from build123d import *

# Parameters (mm, degrees)
F1_DEPTH      = 210
F0_W          = 7
F0_H          = 48
F2_DEPTH      = 202
F5_D          = 2.6
F5_DEPTH      = 8
F5_TIP        = 0.7811188047
F6_D          = 2.6
F6_DEPTH      = 8
F6_TIP        = 0.7811188047
F9_D          = 2.6
F9_DEPTH      = 6
F9_TIP        = 0.7811188047
F10_D         = 2.6
F10_DEPTH     = 15
F10_TIP       = 0.7811188047
F11_W         = 61
F11_H         = 28
F12_DEPTH     = 12.5
F15_D         = 3
F17_D         = 11
F17_DEPTH     = 5
F17_TIP       = 3.3047334047
F18_D         = 11
F18_DEPTH     = 5
F18_TIP       = 3.3047334047
F19_SIZE      = 1
F20_W         = 65
F20_H         = 34
F20_W_2       = 61
F20_H_2       = 28
F21_DEPTH     = 10
F22_R         = 2
F23_T1_DEPTH  = 10
F23_T6_DEPTH  = 10
F23_S7_R      = 1.3
F23_T8_DEPTH  = 7
F23_T12_DEPTH = 10
F23_S13_R     = 1.3
F23_T14_DEPTH = 7
F20_W_3       = 150
F20_H_3       = 44
F24_DEPTH     = 10
F25_R         = 4
F20_W_4       = 34
F20_H_4       = 43.9752993435
F26_DEPTH     = 10
F27_R         = 4


# Not quite as in the source:
# - a fillet or chamfer that OpenCascade refuses, or shapes differently, is made with other operations: its cross-section is extruded or revolved along the edge and cut away or added
# - a feature names something its author has since deleted; it is built from what else it names


with BuildPart() as f1:
    # F0 (on Right) → F1 (new body, symmetric)
    with BuildSketch(Plane.YZ):
        Polygon((3.25, 30), (-3.25, 30), (-3.25, 24), (-3.25, -24), (-3.25, -30), (3.25, -30), align=None)
    extrude(amount=F1_DEPTH, both=True)

    # F0 (on Right) → F2 (join, symmetric)
    with BuildSketch(Plane.YZ):
        Polygon((3.25, 30), (-3.25, 30), (-3.25, 24), (-3.25, -24), (-3.25, -30), (3.25, -30), align=None)
        with Locations((-6.75, 0)):
            Rectangle(F0_W, F0_H)
    extrude(amount=F2_DEPTH, both=True)

    # F5
    with Locations(Plane.XY.offset(24)):
        with Locations((0, -7.25), (-160, -7.25), (160, -7.25)):
            Hole(F5_D / 2, depth=F5_DEPTH)
            with Locations((0, 0, -(F5_DEPTH + F5_TIP / 2))):  # 118° drill point
                Cone(0, F5_D / 2, F5_TIP, mode=Mode.SUBTRACT)

    # F6
    with Locations(Plane(origin=(0, 0, -24), x_dir=(1, 0, 0), z_dir=(0, 0, -1))):
        with Locations((-160, 7.25), (0, 7.25), (160, 7.25)):
            Hole(F6_D / 2, depth=F6_DEPTH)
            with Locations((0, 0, -(F6_DEPTH + F6_TIP / 2))):  # 118° drill point
                Cone(0, F6_D / 2, F6_TIP, mode=Mode.SUBTRACT)

    # F9
    with Locations(Plane(origin=(-202, 0, 0), x_dir=(0, -1, 0), z_dir=(-1, 0, 0))):
        with Locations((7.25, -14), (7.25, 14)):
            Hole(F9_D / 2, depth=F9_DEPTH)
            with Locations((0, 0, -(F9_DEPTH + F9_TIP / 2))):  # 118° drill point
                Cone(0, F9_D / 2, F9_TIP, mode=Mode.SUBTRACT)

    # F10
    with Locations(Plane.YZ.offset(202)):
        with Locations((-7.25, -14), (-7.25, 14)):
            Hole(F10_D / 2, depth=F10_DEPTH)
            with Locations((0, 0, -(F10_DEPTH + F10_TIP / 2))):  # 118° drill point
                Cone(0, F10_D / 2, F10_TIP, mode=Mode.SUBTRACT)


with BuildPart() as f12:
    # F11 (on Front) → F12 (new body, symmetric)
    with BuildSketch(Plane.XZ):
        with Locations((-164.5, 0)):
            Rectangle(F11_W, F11_H)
    extrude(amount=F12_DEPTH, both=True)


with BuildPart() as f1_1:
    add(f1.part)

    # F13: cut F12
    add(f12.part, mode=Mode.SUBTRACT)

    # F15 (through all)
    with Locations(Plane(origin=(0, 3.25, 0), x_dir=(-1, 0, 0), z_dir=(0, 1, 0))):
        with Locations((164.5, 20), (164.5, -20)):
            Hole(F15_D / 2)

    # F17
    with Locations(Plane(origin=(0, 3.25, 0), x_dir=(-1, 0, 0), z_dir=(0, 1, 0))):
        with Locations((-190, 17), (-170, 17), (-170, 0), (-190, 0), (-75.4730241728, 9.8040188106), (-55.4730241728, 9.8040188106), (-75.4730241728, -9.8040188106), (-55.4730241728, -9.8040188106), (-170, -17), (-190, -17), (-35.4730241728, 9.8040188106), (-15.4730241728, 9.8040188106), (-15.4730241728, -9.8040188106), (-35.4730241728, -9.8040188106), (-150, 17), (-130, 17), (-130, 0), (-150, 0), (-150, -17), (-130, -17)):
            Hole(F17_D / 2, depth=F17_DEPTH)
            with Locations((0, 0, -(F17_DEPTH + F17_TIP / 2))):  # 118° drill point
                Cone(0, F17_D / 2, F17_TIP, mode=Mode.SUBTRACT)

    # F18
    with Locations(Plane(origin=(0, 3.25, 0), x_dir=(-1, 0, 0), z_dir=(0, 1, 0))):
        with Locations((-95.4730241728, -9.8040188106), (-95.4730241728, 9.8040188106)):
            Hole(F18_D / 2, depth=F18_DEPTH)
            with Locations((0, 0, -(F18_DEPTH + F18_TIP / 2))):  # 118° drill point
                Cone(0, F18_D / 2, F18_TIP, mode=Mode.SUBTRACT)

    # F19
    f19_edges = [f1_1.edges().sort_by_distance(p)[0] for p in [
        (210, 0, 30),
        (0, 3.25, 30),
        (210, 3.25, 0),
        (0, 3.25, -30),
        (-210, 3.25, 0),
        (-210, 0, 30),
        (-210, 0, -30),
        (210, 0, -30),
    ]]
    chamfer(f19_edges, length=F19_SIZE)

    # F20 (on face) → F21 (cut, symmetric)
    with BuildSketch(Plane.XZ.offset(10.25)):
        with Locations((-164.5, 0)):
            Rectangle(F20_W, F20_H)
        with Locations((-164.5, 0)):
            Rectangle(F20_W_2, F20_H_2, mode=Mode.SUBTRACT)
    extrude(amount=F21_DEPTH, both=True, mode=Mode.SUBTRACT)

    # F22
    f22_edges = [f1_1.edges().sort_by_distance(p)[0] for p in [
        (-195, 1.5, 14),
        (-134, 1.5, 14),
        (-195, 1.5, -14),
        (-134, 1.5, -14),
    ]]
    fillet(f22_edges, radius=F22_R)

    # F23: fillet of radius 4 on 4 edges, made by hand

    # F23_s2 → F23_t1 (join)
    with BuildSketch(Plane.XZ.offset(0.25)):
        with BuildLine():
            ThreePointArc((-136, 17), (-133.1715728753, 15.8284271247), (-132, 13))
            Line((-132, 13), (-132, 17))
            Line((-132, 17), (-136, 17))
        make_face()
        with BuildLine():
            ThreePointArc((-136, -17), (-133.1715728753, -15.8284271247), (-132, -13))
            Line((-132, -13), (-132, -17))
            Line((-132, -17), (-136, -17))
        make_face()
    extrude(amount=F23_T1_DEPTH)


with BuildPart() as f23_tool4:
    # F23_s5 → F23_t6 (new body)
    with BuildSketch(Plane.XZ.offset(0.25)):
        with BuildLine():
            ThreePointArc((-193, 17), (-195.8284271247, 15.8284271247), (-197, 13))
            Line((-197, 13), (-197, 17))
            Line((-197, 17), (-193, 17))
        make_face()
    extrude(amount=F23_T6_DEPTH)

    # F23_s7 → F23_t8 (cut, symmetric)
    with BuildSketch(Plane.YZ.offset(-195)):
        with Locations((-7.25, 14)):
            Circle(F23_S7_R)
    extrude(amount=F23_T8_DEPTH, both=True, mode=Mode.SUBTRACT)


with BuildPart() as f1_2:
    add(f1_1.part)

    # F23_t3: union F23_tool4
    add(f23_tool4.part)


with BuildPart() as f23_tool10:
    # F23_s11 → F23_t12 (new body)
    with BuildSketch(Plane.XZ.offset(0.25)):
        with BuildLine():
            ThreePointArc((-197, -13), (-195.8284271247, -15.8284271247), (-193, -17))
            Line((-193, -17), (-197, -17))
            Line((-197, -17), (-197, -13))
        make_face()
    extrude(amount=F23_T12_DEPTH)

    # F23_s13 → F23_t14 (cut, symmetric)
    with BuildSketch(Plane.YZ.offset(-195)):
        with Locations((-7.25, -14)):
            Circle(F23_S13_R)
    extrude(amount=F23_T14_DEPTH, both=True, mode=Mode.SUBTRACT)


with BuildPart() as f1_3:
    add(f1_2.part)

    # F23_t9: union F23_tool10
    add(f23_tool10.part)

    # F20 (on face) → F24 (cut, symmetric)
    with BuildSketch(Plane.XZ.offset(10.25)):
        with Locations((82, 0)):
            Rectangle(F20_W_3, F20_H_3)
    extrude(amount=F24_DEPTH, both=True, mode=Mode.SUBTRACT)

    # F25
    f25_edges = [f1_3.edges().sort_by_distance(p)[0] for p in [
        (157, -5.25, 22),
        (157, -5.25, -22),
        (7, -5.25, -22),
        (7, -5.25, 22),
    ]]
    fillet(f25_edges, radius=F25_R)

    # F20 (on face) → F26 (cut, symmetric)
    with BuildSketch(Plane.XZ.offset(10.25)):
        with Locations((180, 0.0123503283)):
            Rectangle(F20_W_4, F20_H_4)
    extrude(amount=F26_DEPTH, both=True, mode=Mode.SUBTRACT)

    # F27
    f27_edges = [f1_3.edges().sort_by_distance(p)[0] for p in [
        (163, -5.25, -21.975299),
        (163, -5.25, 22),
        (197, -5.25, 22),
        (197, -5.25, -21.975299),
    ]]
    fillet(f27_edges, radius=F27_R)


solid = f1_3.part
Check sheet for the modelled part. Datum: model origin and axes. Units: mm. A direction names the side the tool comes from. Coordinates: 2 decimals unless noted, no trailing zeros. Write each loop counter-clockwise with the first axis right and the second up, starting at its lowest first coordinate (ties: lowest second). Pieces come first, ordered by that corner, then holes.
Item 1: Access from +Z, -Z, +X, -X, +Y, -Y to the whole of each face (thin tool, end or side, straight path). Record for faces 5 (the face through (148.81, 1.27, -22.37)), 6 (the face through (-202, -7, 0)), 7 (the face through (-167, -0.25, 15)).
Numbers:
face 5: +Y
face 6: +Z, -Z, -X, -Y
face 7: -Y
Item 2: Scan lines: probe 1 along X at (y, z) = (-7.25, -18.25); probe 2 along X at (y, z) = (-4.5, -8.5); probe 3 along Z at (x, y) = (150, 1.5). Record each from-to range of solid material in increasing order.
Numbers:
probe 1: x = -202 to -161.3, -158.7 to -1.3, 1.3 to 7.01, 156.99 to 158.7, 161.3 to 163.01, 196.99 to 202
probe 2: x = -202 to -197, -132 to 7, 157 to 163, 197 to 202
probe 3: z = -30 to -22.5, -11.5 to -5.5, 5.5 to 11.5, 22.5 to 30
Item 3: Cross-section at A-A on x = 57. Record the boundary of the cut face in (y, z).
Numbers:
outline: (-10.25, -24) - (-3.25, -24) - (-3.25, -30) - (2.25, -30) - (3.25, -29) - (3.25, -15.09) - (-0.25, -15.09) - (-0.25, -22) - (-10.25, -22) - close; (-10.25, 22) - (-0.25, 22) - (-0.25, 15.09) - (3.25, 15.09) - (3.25, 29) - (2.25, 30) - (-3.25, 30) - (-3.25, 24) - (-10.25, 24) - close; (-0.25, -4.52) - (3.25, -4.52) - (3.25, 4.52) - (-0.25, 4.52) - close
Item 4: Depth check by flat-ended pin: pin 1 Ø4 at (y, z) = (-7, -5.5) entering from +X; pin 2 Ø5 at (y, z) = (-6.5, -4.5) entering from -X; pin 3 Ø8 at (y, z) = (-6.5, -6.5) entering from -X; pin 4 Ø4 at (x, y) = (160, -7.25) entering from +Z. Enter the tip coordinate at first touch or a pass-through.
Numbers:
pin 1: stops at x = 202
pin 2: stops at x = -202
pin 3: stops at x = -210
pin 4: stops at z = 24
Item 5: Mould release check, pull along Z, two halves, no side actions. Record for faces 1 (the face through (180, -5, -21.975)), 2 (the face through (3, 3.25, 0)), 3 (the face through (3, -7, 24)), 4 (the face through (189.284, 1.271, 22.453)): released by +Z, released by -Z, zero draft, split by the parting line, or undercut.
Numbers:
face 1: undercut
face 2: zero draft
face 3: released by +Z
face 4: undercut
Item 6: Cross-section at B-B on z = 0. Count the separate pieces of the cut face and the enclosed holes in it, then the cut area to 3 significant figures.
Numbers:
separate pieces: 6
enclosed holes: 0
area: 2,700 mm2
